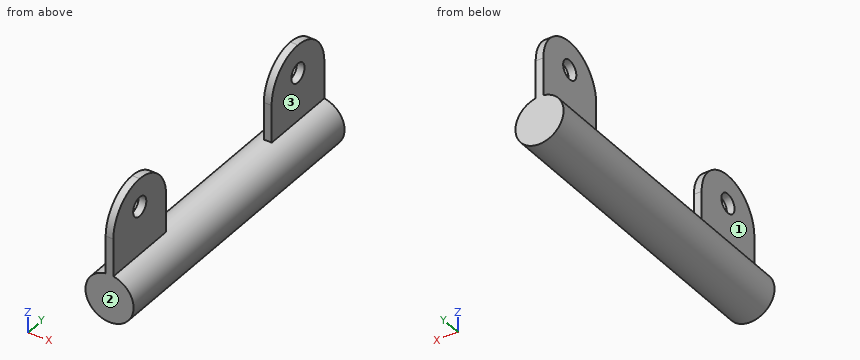
from build123d import *

# Parameters (mm, degrees)
SKETCH1_R            = 12.5
BOSS_EXTRUDE1_DEPTH  = 160
SKETCH2_W            = 4
SKETCH2_H            = 40
BOSS_EXTRUDE2_DEPTH  = 40
FILLET1_R            = 20
SKETCH3_R            = 5
CUT_EXTRUDE1_DEPTH   = 169.861629745
FILLET1_OF_MIRROR2_R = 20


with BuildPart() as part:
    # Sketch1 → Boss-Extrude1 (new body)
    with BuildSketch(Plane(origin=(0, 0, 0), x_dir=(1, 0, 0), z_dir=(0, 1, 0))):
        with Locations(Location((0, 0, 0), (0, 0, 270))):
            Circle(SKETCH1_R)
    extrude(amount=BOSS_EXTRUDE1_DEPTH)

    # Sketch2 → Boss-Extrude2 (add)
    with BuildSketch(Plane.XY.offset(12)):
        with Locations((0, 140)):
            Rectangle(SKETCH2_W, SKETCH2_H)
    boss_extrude2 = extrude(amount=BOSS_EXTRUDE2_DEPTH)

    # Fillet1
    fillet1_edges = [part.edges().sort_by_distance(p)[0] for p in [
        (0, 120, 52),
        (0, 160, 52),
    ]]
    fillet(fillet1_edges, radius=FILLET1_R - 0.0001)  # a hair under: the kernel refuses the full size

    # Sketch3 → Cut-Extrude1 (cut, through all)
    with BuildSketch(Plane(origin=(2, 0, 0), x_dir=(0, 0, -1), z_dir=(1, 0, 0))):
        with Locations(Location((-37.338962679, 140, 0), (0, 0, 90))):
            Circle(SKETCH3_R)
    cut_extrude1 = extrude(amount=-CUT_EXTRUDE1_DEPTH, mode=Mode.SUBTRACT)

    # Mirror2: Boss-Extrude2, Cut-Extrude1 across plane
    add(boss_extrude2.mirror(Plane.ZX.offset(80)))
    add(cut_extrude1.mirror(Plane.ZX.offset(80)), mode=Mode.SUBTRACT)

    # Fillet1 of Mirror2
    fillet1_of_mirror2_edges = [part.edges().sort_by_distance(p)[0] for p in [
        (0, 40, 52),
        (0, 0, 52),
    ]]
    fillet(fillet1_of_mirror2_edges, radius=FILLET1_OF_MIRROR2_R - 0.0001)  # a hair under: the kernel refuses the full size


solid = part.part
For this review, take the finished solid that the model builds, in its own axes (mm). Face numbers are marked on the shaded views. A direction names the side the tool comes from. Coordinates: 2 decimals unless noted, no trailing zeros. Loops run counter-clockwise (first coordinate to the right, second up) from the corner with the lowest first, then second, coordinate; pieces in that order, holes last. Notation, with made-up numbers: (4, 78.5) - (25, 78.5) arc R20 ccw to (25, 97.5) - close; hole circle Ø11 at (-31, 52.5). An arc over 180 degrees is marked (long way). Use a Markdown table: item, result. Add a question column.
Item 1: We need section A-A (z = 25). Give the boundary of the cut face in (x, y).
Item 2: Tool access review of the marked faces 1, 2 and 3: name each direction out of +Z, -Z, +X, -X, +Y, -Y from which nothing blocks a thin tool from reaching the whole face with its end or side.
Item 3: We need section C-C (y = 94). Give the boundary of the cut face in (x, z), and give its area (3 significant figures).
Item 4: For line 1 (Z direction, x = 0.05, y = 140); line 2 (X direction, y = 13, z = 26.5); line 3 (Z direction, x = -2.75, y = 91), list the stretches that pass through material, from the lowest coordinate up.
Item 5: We need section D-D (x = 8.5). Give the boundary of the cut face in (y, z), and give its area (3 significant figures).
Item 6: We need section B-B (x = 0). Give the number of separate pieces and of enclosed holes in the cut face, and give its area (3 significant figures).
Item 7: Insertion check: pin 1 Ø12 at (y, z) = (12.5, 31) entering from +X; pin 2 Ø16 at (y, z) = (20, 37.34) entering from -X; pin 3 Ø2 at (x, y) = (-6, 114.5) entering from -Z; pin 4 Ø8 at (y, z) = (140, 37.34) entering from +X. Each pin has a flat end and moves straight along its axis. Give the tip position at first contact, or say it passes through.
Results list:
| question | item | result |
|---|---|---|
| 1 | outline | (-2, 0) - (2, 0) - (2, 40) - (-2, 40) - close; (-2, 120) - (2, 120) - (2, 160) - (-2, 160) - close |
| 2 | face 1 | +Z, -X, +Y, -Y |
| 2 | face 2 | +Z, -Z, +X, -X, -Y |
| 2 | face 3 | +Z, +X, +Y, -Y |
| 3 | outline | circle Ø25 at (0, 0) |
| 3 | area | 491 mm^2 |
| 4 | line 1 | z = -12.5 to 32.34, 42.34 to 52 |
| 4 | line 2 | x = -2 to 2 |
| 4 | line 3 | z = -12.19 to 12.19 |
| 5 | outline | (0, -9.17) - (160, -9.17) - (160, 9.17) - (0, 9.17) - close |
| 5 | area | 2,930 mm^2 |
| 6 | separate pieces | 1 |
| 6 | enclosed holes | 2 |
| 6 | area | 6,660 mm^2 |
| 7 | pin 1 | stops at x = 2 |
| 7 | pin 2 | stops at x = -2 |
| 7 | pin 3 | stops at z = -11.46 |
| 7 | pin 4 | passes through |
